```python
from build123d import *

# Parameters (mm, degrees)
SKETCH1_W           = 56.55
SKETCH1_H           = 12.7
BOSS_EXTRUDE1_DEPTH = 33
SKETCH2_R           = 1.5
CUT_EXTRUDE1_DEPTH  = 10
CUT_EXTRUDE2_DEPTH  = 66.781646376


with BuildPart() as part:
    # Sketch1 → Boss-Extrude1 (new body)
    with BuildSketch(Plane.XY):
        Rectangle(SKETCH1_W, SKETCH1_H)
    extrude(amount=BOSS_EXTRUDE1_DEPTH)

    # Sketch2 → Cut-Extrude1 (cut)
    with BuildSketch(Plane.XY.offset(33)):
        with BuildLine():
            Line((-20.5, 0), (-17.5, 0))
            Line((-17.5, 0), (-14.5, 0))
            ThreePointArc((-14.5, 0), (-17.5, 3), (-20.5, 0))
        make_face()
        with BuildLine():
            Line((-14.5, 0), (-17.5, 0))
            Line((-17.5, 0), (-20.5, 0))
            ThreePointArc((-20.5, 0), (-17.5, -3), (-14.5, 0))
        make_face()
        with BuildLine():
            ThreePointArc((20.5, 0), (17.5, 3), (14.5, 0))
            Line((14.5, 0), (17.5, 0))
            Line((17.5, 0), (20.5, 0))
        make_face()
        with BuildLine():
            Line((17.5, 0), (14.5, 0))
            ThreePointArc((14.5, 0), (17.5, -3), (20.5, 0))
            Line((20.5, 0), (17.5, 0))
        make_face()
        Circle(SKETCH2_R)
    extrude(amount=-CUT_EXTRUDE1_DEPTH, mode=Mode.SUBTRACT)

    # Sketch3 → Cut-Extrude2 (cut, through all)
    with BuildSketch(Plane.ZY.offset(28.275)):
        with BuildLine():
            ThreePointArc((5.5, 0), (7, -1.5), (8.5, 0))
            Line((8.5, 0), (5.5, 0))
        make_face()
        with BuildLine():
            Line((5.5, 0), (8.5, 0))
            ThreePointArc((8.5, 0), (7, 1.5), (5.5, 0))
        make_face()
        with BuildLine():
            ThreePointArc((15.5, 0), (17, -1.5), (18.5, 0))
            Line((18.5, 0), (15.5, 0))
        make_face()
        with BuildLine():
            Line((15.5, 0), (18.5, 0))
            ThreePointArc((18.5, 0), (17, 1.5), (15.5, 0))
        make_face()
    extrude(amount=-CUT_EXTRUDE2_DEPTH, mode=Mode.SUBTRACT)


solid = part.part
```
Work out the finished part from the listing and answer in its coordinate system (mm). A direction names the side the tool comes from. Coordinates: 2 decimals unless noted, no trailing zeros. Loops run counter-clockwise (first coordinate to the right, second up) from the corner with the lowest first, then second, coordinate; pieces in that order, holes last.
1) For a pull along Z with two mould halves and no side action, classify faces 3 (the flat face through (28.275, -2, 16)), 4 (the flat face through (17, 0, 23)), 5 (the cylindrical face through (-0.4, 0.07, 15.5)) as +Z half, -Z half, draft (parallel to the pull), parting line (faces both ways), or undercut.
Results:
face 3: draft
face 4: +Z half
face 5: undercut
2) Section A-A (z = 28.5) is taken. Give the vertices of the cut face in (x, y) (3 decimals), plus the area to 3 significant figures.
Results:
outline: (-28.275, -6.35) - (28.275, -6.35) - (28.275, 6.35) - (-28.275, 6.35) - close; hole circle Ø6 at (-17.5, 0); hole circle Ø3 at (0, 0); hole circle Ø6 at (17.5, 0)
area: 655 mm2
3) For faces 1 (the cylindrical face through (-1.5, 0.07, 28.07)), 2 (the flat face through (-28.275, -2, 16)), determine the directions among +Z, -Z, +X, -X, +Y, -Y from which every point of the face is accessible in a straight line to the end or side of a thin tool.
Results:
face 1: +Z
face 2: +Z, -Z, -X, +Y, -Y
4) Section C-C (z = 17) is taken. Give the vertices of the cut face in (x, y) (3 decimals), plus the area to 3 significant figures.
Results:
outline: (-28.275, -6.35) - (28.275, -6.35) - (28.275, -1.5) - (-28.275, -1.5) - close; (-28.275, 1.5) - (28.275, 1.5) - (28.275, 6.35) - (-28.275, 6.35) - close
area: 549 mm2
5) Consider probe 1 along Y at (x, z) = (-5, 7); probe 2 along X at (y, z) = (2.75, 28.5) (3 decimals); probe 3 along X at (y, z) = (2.25, 28) (3 decimals). Determine where each line is inside the solid, lowest interval first.
Results:
probe 1: y = -6.35 to -1.5, 1.5 to 6.35
probe 2: x = -28.275 to -18.699, -16.301 to 16.301, 18.699 to 28.275
probe 3: x = -28.275 to -19.484, -15.516 to 15.516, 19.484 to 28.275
6) Section B-B (y = 0) is taken. Give the vertices of the cut face in (x, z) (3 decimals), plus the area to 3 significant figures.
Results:
outline: (-28.275, 0) - (28.275, 0) - (28.275, 5.5) - (-28.275, 5.5) - close; (-28.275, 8.5) - (28.275, 8.5) - (28.275, 15.5) - (-28.275, 15.5) - close; (-28.275, 18.5) - (28.275, 18.5) - (28.275, 33) - (20.5, 33) - (20.5, 23) - (14.5, 23) - (14.5, 33) - (1.5, 33) - (1.5, 23) - (-1.5, 23) - (-1.5, 33) - (-14.5, 33) - (-14.5, 23) - (-20.5, 23) - (-20.5, 33) - (-28.275, 33) - close
area: 1,380 mm2
7) A flat-ended cylindrical pin translates along its axis: pin 1 (3.5 mm diameter, centred on x = 17.5, y = 0, fed in from +Z). Find the tip coordinate at first contact, or state that the pin passes through.
Results:
pin 1: stops at z = 23
8) Section D-D (x = -3) is taken. Give the vertices of the cut face in (y, z), plus the area to 3 significant figures.
Results:
outline: (-6.35, 0) - (6.35, 0) - (6.35, 33) - (-6.35, 33) - close; hole circle Ø3 at (0, 7); hole circle Ø3 at (0, 17)
area: 405 mm2
